For this review, take the finished solid that the model builds, in its own axes (mm). A direction names the side the tool comes from. Give positions to 0.01 mm unless a question says otherwise; leave off trailing zeros. Loops run counter-clockwise (first coordinate to the right, second up) from the corner with the lowest first, then second, coordinate; pieces in that order, holes last. Notation, with made-up numbers: (27.5, -28.75) -> (68.5, -28.75) arc R22 cw to (68.5, -15.75) -> close; hole circle Ø2 at (71.5, -37.75). An arc over 180 degrees is marked (long way). One line per question, with ' | ' between items. Start each with the question number.
(1) Wall thickness on probe 1 along X at (y, z) = (6.5, 1) (3 decimals); probe 2 along X at (y, z) = (4, -2) (3 decimals); probe 3 along Y at (x, z) = (11, 2): over which ranges is each line inside the solid? List them lowest first.
(2) Draft analysis for pull direction Z (two halves, no side actions). For faces 1 (the cylindrical face through (24.631, 1.717, 2.664)), 2 (the flat face through (0, 0, 0)), 3 (the conical face through (20.4, 0.5, 0.1)), 4 (the conical face through (-20.4, 0.5, 0.1)), state which applies: +Z half, -Z half, draft (parallel to the pull), parting line (faces both ways), or undercut.
(3) Insertion check: P1, Ø2.5, axis at x = 13.76, y = 3.39, coming from the +Z side; P2, Ø1.3, axis at y = 5, z = 0.5, coming from the -X side (3 decimals). Each pin has a flat end and moves straight along its axis. Give the tip position at first contact, or say it passes through.
(4) Consider section C-C (y = 2.75). Give the number of separate pieces and of enclosed holes in the cut face, and give its area (3 significant figures).
(5) Consider section B-B (x = -6). Write out the cut boundary in (y, z), and give its area (3 significant figures).
(6) Tool access review of faces 5 (the flat face through (-18.5, 3.386, 0.1)), 6 (the cylindrical face through (-24.631, 1.669, 2.664)), 7 (the flat face through (18.6, 3.386, -0.8)): name each direction out of +Z, -Z, +X, -X, +Y, -Y from which nothing blocks a thin tool from reaching the whole face with its end or side.
(7) Consider section A-A (y = 8.25). Write out the cut boundary in (x, z), and give its area (3 significant figures).
from build123d import *

# Parameters (mm, degrees)
F1_DEPTH = 3.81
F3_R     = 3.80999
F4_R     = 2.54
F2_R     = 1.905
F5_DEPTH = 3.81


# Not quite as in the source:
# - a fillet or chamfer is up to 0.001 mm smaller than in the source, because OpenCascade refuses the exact size
# - a pattern or mirror of a feature is missing from the dataset's text; its kind, count and spacing are read off the source's solid


with BuildPart() as f1:
    # F0 (on Top) → F1 (new body, symmetric)
    with BuildSketch(Plane.XY):
        Polygon((17.145, 10.16), (0, 10.16), (-17.145, 10.16), (-17.145, 3.38582), (-25.7175, 3.38582), (-25.7175, 0), (0, 0), (25.7175, 0), (25.7175, 3.38582), (17.145, 3.38582), align=None)
    extrude(amount=F1_DEPTH, both=True)

    # F3 (radius 3.81 in the source; OpenCascade refuses exactly that, so slightly less here)
    f3_edges = [f1.edges().sort_by_distance(p)[0] for p in [
        (-25.7175, 1.69291, 3.81),
        (-25.7175, 1.69291, -3.81),
        (25.7175, 1.69291, 3.81),
        (25.7175, 1.69291, -3.81),
    ]]
    fillet(f3_edges, radius=F3_R)

    # F4
    f4_edges = [f1.edges().sort_by_distance(p)[0] for p in [
        (-17.145, 10.16, 0),
        (17.145, 10.16, 0),
    ]]
    fillet(f4_edges, radius=F4_R)

    # F2 (on Top) → F5 (cut, symmetric)
    with BuildSketch(Plane.XY):
        with Locations((-13.7583333333, 6.7733333333)):
            Circle(F2_R)
        with Locations((-10.3716666667, 3.3866666667)):
            Circle(F2_R)
        with Locations((-2.3283333333, 3.3866666667)):
            Circle(F2_R)
        with Locations((-5.715, 6.7733333333)):
            Circle(F2_R)
        with Locations((5.715, 3.3866666667)):
            Circle(F2_R)
        with Locations((2.3283333333, 6.7733333333)):
            Circle(F2_R)
        with Locations((13.7583333333, 3.3866666667)):
            Circle(F2_R)
        with Locations((10.3716666667, 6.7733333333)):
            Circle(F2_R)
    extrude(amount=F5_DEPTH, both=True, mode=Mode.SUBTRACT)

    # F6 (on Top) → F7 (revolve, cut)
    with BuildSketch(Plane.XY):
        Polygon((-21.9075, -2.113441314), (-21.9075, 3.38582), (-25.0825, 3.38582), align=None)
    f7 = revolve(axis=Axis((-21.9075, 0.636189343, 0), (0, 1, 0)), mode=Mode.SUBTRACT)

    # F7_copies: F7 across plane
    add(f7.mirror(Plane(origin=(0, 0, 0), x_dir=(0, 0, 1), z_dir=(1, 0, 0))), mode=Mode.SUBTRACT)


solid = f1.part
A:
1) probe 1: x = -17.145 to -15.644, -11.873 to -7.6, -3.83 to 0.443, 4.214 to 8.486, 12.257 to 17.145 | probe 2: x = -17.145 to -12.175, -8.568 to -4.132, -0.525 to 3.911, 7.519 to 11.955, 15.562 to 17.145 | probe 3: y = 0 to 4.97, 8.57 to 10.16
2) face 1: +Z half | face 2: draft | face 3: undercut | face 4: undercut
3) P1: passes through | P2: stops at x = -17.145
4) separate pieces: 5 | enclosed holes: 2 | area: 220 mm^2
5) outline: (0, -3.81) -> (4.89, -3.81) -> (4.89, 3.81) -> (0, 3.81) -> close; (8.66, -3.81) -> (10.16, -3.81) -> (10.16, 3.81) -> (8.66, 3.81) -> close | area: 48.7 mm^2
6) face 5: +Z, -Z, -X, +Y | face 6: +Z, -X, +Y, -Y | face 7: +Z, -Z, +X, +Y
7) outline: (-17.07, -3.81) -> (-14.96, -3.81) -> (-14.96, 3.81) -> (-17.07, 3.81) -> close; (-12.55, -3.81) -> (-6.92, -3.81) -> (-6.92, 3.81) -> (-12.55, 3.81) -> close; (-4.51, -3.81) -> (1.12, -3.81) -> (1.12, 3.81) -> (-4.51, 3.81) -> close; (3.53, -3.81) -> (9.17, -3.81) -> (9.17, 3.81) -> (3.53, 3.81) -> close; (11.58, -3.81) -> (17.07, -3.81) -> (17.07, 3.81) -> (11.58, 3.81) -> close | area: 187 mm^2
